Source: three-view drawing plus pictorial views. Frame: mm from the lowest corner of the part. A direction names the side the tool comes from. Give positions to 0.01 mm unless a question says otherwise; leave off trailing zeros. Order: outer loops, then holes, each group sorted by start corner. A loop starts at its lowest first (then second) coordinate and runs counter-clockwise, first axis right, second up. Notation, with made-up numbers: M 25,64.25 L 81,64.25 A16 cw 81,73.25 Z; hole C 21.5,36.25 d7. An arc over 180 degrees is marked long. Use CSV: the item, a comma, the result in double quotes. Start each with the question number.
1. Line query: line 1 along X through (y, z) = (5, 7.7); line 2 along Y through (x, z) = (5, 6.7); line 3 along X through (y, z) = (0.5, 4). Output: solid intervals per line, ascending. Write a range as [from, to].
2. Section query D-D, the plane z = 3. Return the cut outline in (x, y).
3. Section query B-B, the plane x = 5. Return the cut outline in (y, z).
4. Mould query, pull axis X, two halves, no side actions, for the marked faces 1, 2, 3 and 4. Classes: released by +X, released by -X, zero draft, split by the parting line, or undercut.
5. Reachability of the marked faces 5, 6 and 7 from +Z, -Z, +X, -X, +Y, -Y: full face, straight path, thin tool, end or side. Return the list, or none.
6. Pin query (flat end, axial travel): P1, Ø1.1, axis at y = 4, z = 4.5, coming from the -X side; P2, Ø2, axis at x = 8.5, y = 6.5, coming from the +Z side; P3, Ø1.5, axis at x = 5.5, y = 8.5, coming from the -Z side. Return the tip coordinate at first contact, or that it passes through.
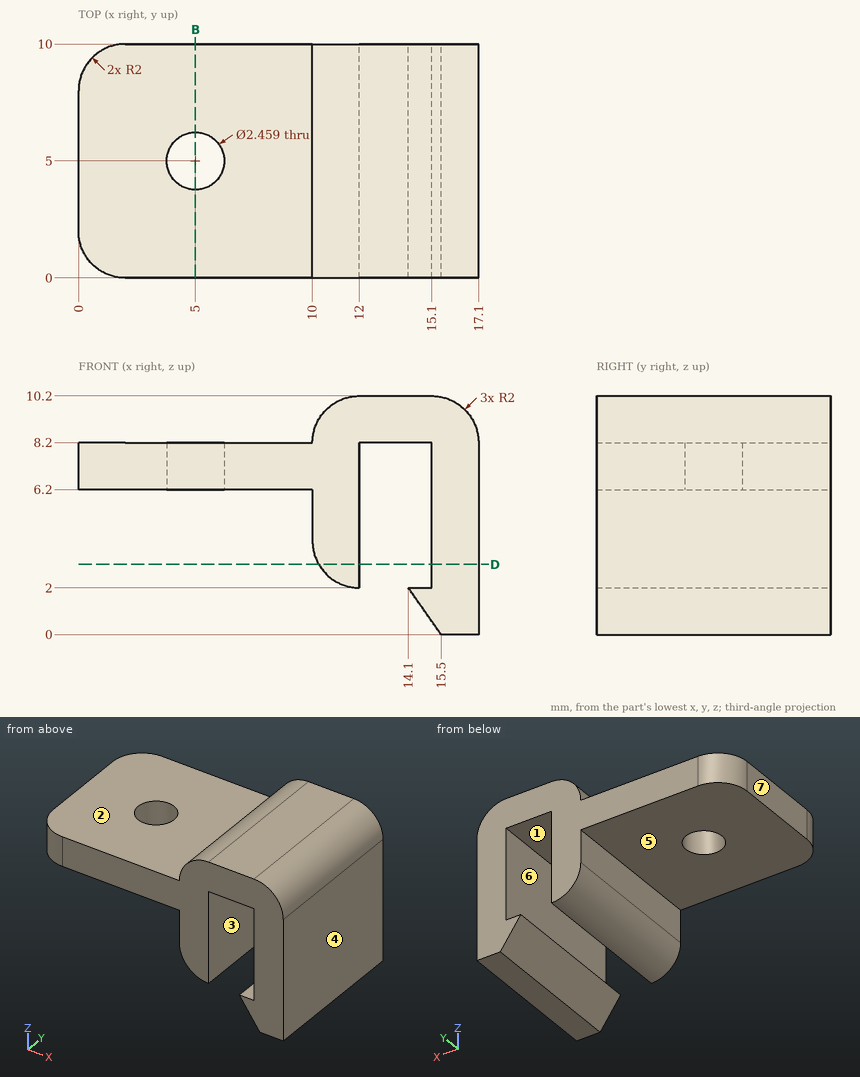
Result set:
1,line 1,"[0, 3.77], [6.23, 12], [15.1, 17.1]"
1,line 2,"[0, 3.77], [6.23, 10]"
1,line 3,"[10, 12], [15.1, 17.1]"
2,outline,"M 10.27,0 L 12,0 L 12,10 L 10.27,10 Z; M 15.1,0 L 17.1,0 L 17.1,10 L 15.1,10 Z"
3,outline,"M 0,6.2 L 3.77,6.2 L 3.77,8.2 L 0,8.2 Z; M 6.23,6.2 L 10,6.2 L 10,8.2 L 6.23,8.2 Z"
4,face 1,"undercut"
4,face 2,"zero draft"
4,face 3,"undercut"
4,face 4,"released by +X"
5,face 5,"-Z, -X, +Y, -Y"
5,face 6,"+Y, -Y"
5,face 7,"+Z, -Z, -X, +Y, -Y"
6,P1,"x = 10"
6,P2,"z = 8.2"
6,P3,"z = 6.2"
